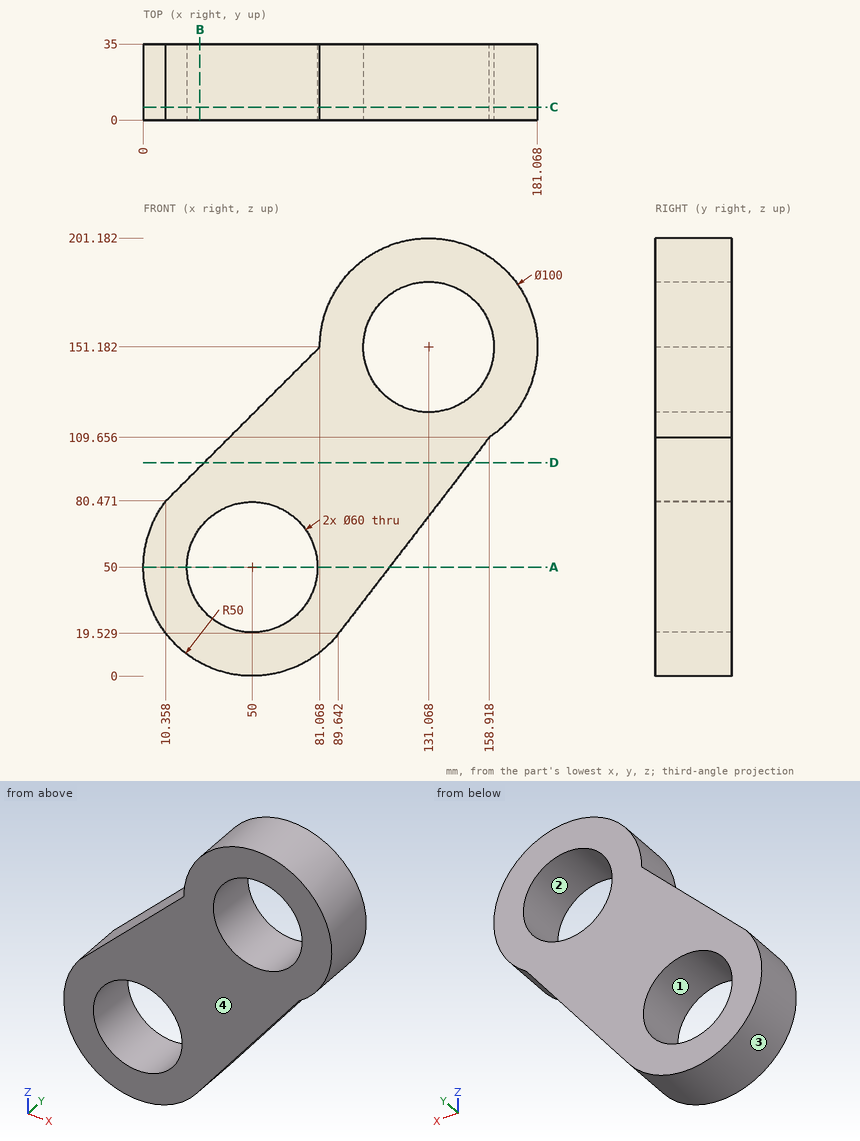
Study the drawing (mm; zero at the part's minimum x, y, z) and answer. Give positions to 0.01 mm unless a question says otherwise; leave off trailing zeros. Order: outer loops, then holes, each group sorted by start corner. A loop starts at its lowest first (then second) coordinate and runs counter-clockwise, first axis right, second up. Notation, with made-up numbers: (55, 26) - (100, 26) arc R21 ccw to (100, 53) - close; hole circle Ø1 at (59, 6). An arc over 180 degrees is marked (long way). Answer in a Markdown table with one row per item. Add a question column.
Q1. The part is cut by section B-B (x = 26). Determine the outline of the cut face in (y, z).
Q2. Given P1, Ø1.5, axis at y = 4.5, z = 65.5, coming from the +X side (1 decimal); P2, Ø4, axis at x = 37, y = 28, coming from the +Z side (1 decimal); P3, Ø3, axis at y = 16.5, z = 28.5, coming from the +X side; P4, Ø8, axis at x = 147.5, z = 98, coming from the -Y side, each flat-ended and moving along its own axis, determine where each tip first touches the part or whether it passes through.
Q3. The part is cut by section A-A (z = 50). Determine the outline of the cut face in (x, y), then the cut area to 3 significant figures.
Q4. Find the intervals of material crossed by line 1 along X through (y, z) = (3, 70.5) (1 decimal); line 2 along X through (y, z) = (32, 37) (1 decimal); line 3 along Z through (x, y) = (50, 20) (1 decimal), in increasing order. Write a range as [from, to].
Q5. The part is cut by section C-C (y = 6). Determine the outline of the cut face in (x, z) (1 decimal), then the cut area to 3 significant figures.
Q6. The part is cut by section D-D (z = 98). Determine the outline of the cut face in (x, y), then the cut area to 3 significant figures.
Q7. For a pull along X with two mould halves and no side action, classify the marked faces 1, 2, 3 and 4 as released by +X, released by -X, zero draft, split by the parting line, or undercut.
Determined:
| question | item | result |
|---|---|---|
| 1 | outline | (0, 6.14) - (35, 6.14) - (35, 32) - (0, 32) - close; (0, 68) - (35, 68) - (35, 96.11) - (0, 96.11) - close |
| 2 | P1 | stops at x = 125.6 |
| 2 | P2 | stops at z = 109.1 |
| 2 | P3 | stops at x = 97.69 |
| 2 | P4 | stops at y = 0 |
| 3 | outline | (0, 0) - (20, 0) - (20, 35) - (0, 35) - close; (80, 0) - (113.06, 0) - (113.06, 35) - (80, 35) - close |
| 3 | area | 1,860 mm² |
| 4 | line 1 | x = [4.4, 28.1], [71.9, 128.8] |
| 4 | line 2 | x = [1.7, 23], [77, 103.1] |
| 4 | line 3 | z = [0, 20], [80, 120.1] |
| 5 | outline | (10.4, 80.5) arc R50 ccw to (89.6, 19.5) - (158.9, 109.7) arc R50 ccw (long way) to (81.1, 151.2) - close; hole circle Ø60 at (50, 50); hole circle Ø60 at (131.1, 151.2) |
| 5 | area | 14,400 mm² |
| 6 | outline | (27.89, 0) - (149.96, 0) - (149.96, 35) - (27.89, 35) - close |
| 6 | area | 4,270 mm² |
| 7 | face 1 | undercut |
| 7 | face 2 | undercut |
| 7 | face 3 | split by the parting line |
| 7 | face 4 | zero draft |
